The model under review builds one solid part; all positions refer to its coordinate system, in mm. Face numbers are marked on the shaded views. A direction names the side the tool comes from. Round coordinates to 2 decimals unless told otherwise and drop trailing zeros. Order: outer loops, then holes, each group sorted by start corner. A loop starts at its lowest first (then second) coordinate and runs counter-clockwise, first axis right, second up. Notation, with made-up numbers: M -16,-1.75 L -8,-1.75 A22 ccw -8,14.25 Z; hole C -16.5,-8.75 d1. An arc over 180 degrees is marked long. Answer as CSV lines item,"result". Start each with the question number.
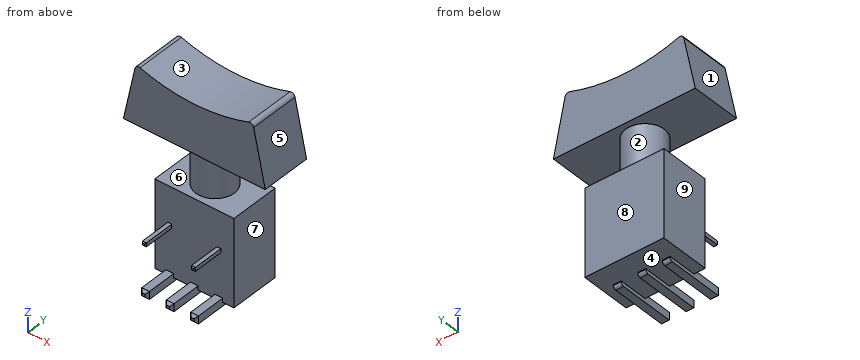
from build123d import *

# Parameters (mm, degrees)
SKETCH1_W           = 8.2
SKETCH1_H           = 9
BOSS_EXTRUDE1_DEPTH = 5.2
SKETCH2_W           = 0.4
SKETCH2_H           = 0.4
SKETCH2_W_2         = 0.8
SKETCH2_H_2         = 0.8
BOSS_EXTRUDE2_DEPTH = 3.3
CHAMFER1_SIZE       = 0.1
CHAMFER2_SIZE       = 0.25
SKETCH2_2_W         = 0.8
SKETCH2_2_H         = 0.38
BOSS_EXTRUDE3_DEPTH = 3
FILLET1_R           = 0.3
SKETCH3_R           = 2
BOSS_EXTRUDE4_DEPTH = 4.5
SKETCH4_W           = 14.7
SKETCH4_H           = 5.2
BOSS_EXTRUDE5_DEPTH = 6.1
CUT_EXTRUDE1_DEPTH  = 19.822393578
FILLET2_R           = 0.4


with BuildPart() as part:
    # Sketch1 → Boss-Extrude1 (new body)
    with BuildSketch(Plane(origin=(0, 0, 0), x_dir=(1, 0, 0), z_dir=(0, 1, 0))):
        Rectangle(SKETCH1_W, SKETCH1_H)
    extrude(amount=BOSS_EXTRUDE1_DEPTH)

    # Sketch2 → Boss-Extrude2 (add)
    with BuildSketch(Plane.XZ):
        with Locations((-2.54, 0.6)):
            Rectangle(SKETCH2_W, SKETCH2_H)
        with Locations((2.54, 0.6)):
            Rectangle(SKETCH2_W, SKETCH2_H)
        with Locations((-2.54, -4.48)):
            Rectangle(SKETCH2_W_2, SKETCH2_H_2)
        with Locations((0, -4.48)):
            Rectangle(SKETCH2_W_2, SKETCH2_H_2)
        with Locations((2.54, -4.48)):
            Rectangle(SKETCH2_W_2, SKETCH2_H_2)
    extrude(amount=BOSS_EXTRUDE2_DEPTH)

    # Chamfer1
    chamfer1_edges = [part.edges().sort_by_distance(p)[0] for p in [
        (-2.34, -3.3, 0.6),
        (-2.54, -3.3, 0.8),
        (-2.74, -3.3, 0.6),
        (-2.54, -3.3, 0.4),
        (2.74, -3.3, 0.6),
        (2.54, -3.3, 0.8),
        (2.34, -3.3, 0.6),
        (2.54, -3.3, 0.4),
    ]]
    chamfer(chamfer1_edges, length=CHAMFER1_SIZE)

    # Chamfer2
    chamfer2_edges = [part.edges().sort_by_distance(p)[0] for p in [
        (-2.14, -3.3, -4.48),
        (-2.54, -3.3, -4.08),
        (-2.94, -3.3, -4.48),
        (-2.54, -3.3, -4.88),
        (0.4, -3.3, -4.48),
        (0, -3.3, -4.08),
        (-0.4, -3.3, -4.48),
        (0, -3.3, -4.88),
        (2.94, -3.3, -4.48),
        (2.54, -3.3, -4.08),
        (2.14, -3.3, -4.48),
        (2.54, -3.3, -4.88),
    ]]
    chamfer(chamfer2_edges, length=CHAMFER2_SIZE)

    # Sketch2<2> → Boss-Extrude3 (add)
    with BuildSketch(Plane.XZ):
        with Locations((-2.54, -4.69)):
            Rectangle(SKETCH2_2_W, SKETCH2_2_H)
        with Locations((0, -4.69)):
            Rectangle(SKETCH2_2_W, SKETCH2_2_H)
        with Locations((2.54, -4.69)):
            Rectangle(SKETCH2_2_W, SKETCH2_2_H)
    extrude(amount=-BOSS_EXTRUDE3_DEPTH)

    # Fillet1
    fillet1_edges = [part.edges().sort_by_distance(p)[0] for p in [
        (-2.54, 3, -4.88),
        (0, 3, -4.88),
        (2.54, 3, -4.88),
    ]]
    fillet(fillet1_edges, radius=FILLET1_R)

    # Sketch3 → Boss-Extrude4 (add)
    with BuildSketch(Plane.XY.offset(4.5)):
        with Locations((0, 2.6)):
            Circle(SKETCH3_R)
    extrude(amount=BOSS_EXTRUDE4_DEPTH)

    # Sketch4 → Boss-Extrude5 (add)
    with BuildSketch(Plane.XY.offset(9)):
        with Locations((0, 2.6)):
            Rectangle(SKETCH4_W, SKETCH4_H)
    extrude(amount=BOSS_EXTRUDE5_DEPTH)

    # Sketch5 → Cut-Extrude1 (cut, through all)
    with BuildSketch(Plane(origin=(0, 5.2, 0), x_dir=(1, 0, 0), z_dir=(0, 1, 0))):
        Polygon((-6.056784937, -15.1), (-7.35, -9), (-7.35, -15.1), align=None)
        with BuildLine():
            ThreePointArc((6.056784937, -15.1), (0, -14.020611804), (-6.056784937, -15.1))
            Line((-6.056784937, -15.1), (6.056784937, -15.1))
        make_face()
        Polygon((7.35, -9), (6.056784937, -15.1), (7.35, -15.1), align=None)
    extrude(amount=-CUT_EXTRUDE1_DEPTH, mode=Mode.SUBTRACT)

    # Fillet2
    fillet2_edges = [part.edges().sort_by_distance(p)[0] for p in [
        (6.056784937, 2.6, 15.1),
        (-6.056784937, 2.6, 15.1),
    ]]
    fillet(fillet2_edges, radius=FILLET2_R)


solid = part.part
Item 1: Consider section D-D (x = -1.25). State the section outline as (y, z) points.
Item 2: Consider section C-C (z = -2.25). State the section outline as (x, y) points, and give its area (3 significant figures).
Item 3: Tool access review of the marked faces 5, 6, 7, 8 and 9: name each direction out of +Z, -Z, +X, -X, +Y, -Y from which nothing blocks a thin tool from reaching the whole face with its end or side.
Item 4: The part is to be moulded in two halves that separate along X. For the marked faces 1, 2, 3 and 4, say which applies: +X half, -X half, draft (parallel to the pull), parting line (faces both ways), or undercut.
Item 5: Consider section B-B (x = -3.75). State the section outline as (y, z) points, and give its area (3 significant figures).
Item 6: Wall thickness on probe 1 along Y at (x, z) = (-2.5, 1.5); probe 2 along Z at (x, y) = (0.25, 2.25); probe 3 along X at (y, z) = (1.25, -1.75): over which ranges is each line inside the solid? List them lowest first. Write a range as [from, to].
Item 7: For pin 1 (1.6 mm diameter, centred on x = 0, y = 1.5, fed in from +Z); pin 2 (5 mm diameter, centred on x = 3, z = 10.5, fed in from -Y); pin 3 (0.6 mm diameter, centred on x = 0, y = -1, fed in from +Z); pin 4 (8 mm diameter, centred on x = 4.5, z = 1.5, fed in from +Y), all flat-tipped, find the tip position at first contact; note any pin that passes through.
Item 8: Consider section A-A (y = -2). State the section outline as (x, z) points.
Reported:
1,outline,"M 0,-4.5 L 5.2,-4.5 L 5.2,4.5 L 4.16,4.5 L 4.16,9 L 5.2,9 L 5.2,14.07 L 0,14.07 L 0,9 L 1.04,9 L 1.04,4.5 L 0,4.5 Z"
2,outline,"M -4.1,0 L 4.1,0 L 4.1,5.2 L -4.1,5.2 Z"
2,area,"42.6 mm²"
3,face 5,"+Z, +X, +Y, -Y"
3,face 6,"none"
3,face 7,"-Z, +X, +Y, -Y"
3,face 8,"+Z, -Z, +X, -X, +Y"
3,face 9,"-Z, -X, +Y, -Y"
4,face 1,"-X half"
4,face 2,"parting line"
4,face 3,"undercut"
4,face 4,"undercut"
5,outline,"M 0,-4.5 L 5.2,-4.5 L 5.2,4.5 L 0,4.5 Z; M 0,9 L 5.2,9 L 5.2,14.43 L 0,14.43 Z"
5,area,"75.0 mm²"
6,probe 1,"y = [0, 5.2]"
6,probe 2,"z = [-4.88, 14.02]"
6,probe 3,"x = [-4.1, 4.1]"
7,pin 1,"stops at z = 14.04"
7,pin 2,"stops at y = 0"
7,pin 3,"stops at z = -4.08"
7,pin 4,"stops at y = 5.2"
8,outline,"M -2.94,-4.88 L -2.14,-4.88 L -2.14,-4.08 L -2.94,-4.08 Z; M -2.74,0.4 L -2.34,0.4 L -2.34,0.8 L -2.74,0.8 Z; M -0.4,-4.88 L 0.4,-4.88 L 0.4,-4.08 L -0.4,-4.08 Z; M 2.14,-4.88 L 2.94,-4.88 L 2.94,-4.08 L 2.14,-4.08 Z; M 2.34,0.4 L 2.74,0.4 L 2.74,0.8 L 2.34,0.8 Z"
